from build123d import *

# Parameters (mm, degrees)
SKETCH_1_R          = 37.15
SKETCH_1_R_2        = 28
SKETCH_1_R_3        = 1.5
EXTRUDE_1_DEPTH     = 3
SKETCH_3_R          = 3
CUT_EXTRUDE_1_DEPTH = 2
CUT_EXTRUDE_START   = -0.5
SKETCH_4_R          = 37.15
CUT_EXTRUDE_2_DEPTH = 0.5


with BuildPart() as part:
    # 草图1 → 凸台-拉伸1 (new body)
    with BuildSketch(Plane(origin=(0, 0, 0), x_dir=(1, 0, 0), z_dir=(0, 1, 0))):
        with Locations(Location((0, 0, 0), (0, 0, 270))):
            Circle(SKETCH_1_R)
        with Locations(Location((0, 0, 0), (0, 0, 270))):
            Circle(SKETCH_1_R_2, mode=Mode.SUBTRACT)
        with Locations(Location((0, 34.825, 0), (0, 0, 270))):
            Circle(SKETCH_1_R_3, mode=Mode.SUBTRACT)
        with Locations(Location((-34.825, 0, 0), (0, 0, 270))):
            Circle(SKETCH_1_R_3, mode=Mode.SUBTRACT)
        with Locations(Location((0, -34.825, 0), (0, 0, 270))):
            Circle(SKETCH_1_R_3, mode=Mode.SUBTRACT)
        with Locations(Location((34.825, 0, 0), (0, 0, 270))):
            Circle(SKETCH_1_R_3, mode=Mode.SUBTRACT)
    extrude(amount=EXTRUDE_1_DEPTH)

    # 草图3 → 切除-拉伸1 (cut)
    with BuildSketch(Plane(origin=(0, 3, 0), x_dir=(1, 0, 0), z_dir=(0, 1, 0))):
        with Locations((0, 34.825)):
            Circle(SKETCH_3_R)
        with Locations((-34.825, 0)):
            Circle(SKETCH_3_R)
        with Locations((0, -34.825)):
            Circle(SKETCH_3_R)
        with Locations((34.825, 0)):
            Circle(SKETCH_3_R)
    extrude(amount=-CUT_EXTRUDE_1_DEPTH, mode=Mode.SUBTRACT)

    # 草图4 → 切除-拉伸2 (cut)
    with BuildSketch(Plane(origin=(0, 3, 0), x_dir=(1, 0, 0), z_dir=(0, 1, 0)).offset(CUT_EXTRUDE_START)):
        with Locations(Location((0, 0, 0), (0, 0, 93.02036647))):
            Circle(SKETCH_4_R)
    extrude(amount=CUT_EXTRUDE_2_DEPTH, mode=Mode.SUBTRACT)


solid = part.part
CAD build for the part. Positions are in the model's coordinates, mm. A direction names the side the tool comes from. Round coordinates to 2 decimals unless told otherwise and drop trailing zeros. Write each loop counter-clockwise with the first axis right and the second up, starting at its lowest first coordinate (ties: lowest second). Pieces come first, ordered by that corner, then holes.
(1) 3-axis set-ups, long thin cutter, end or side, ignore diameter. For faces 4 (the face through (0, 1, 33)), 5 (the face through (24, 2.5, -15)): which of +Z, -Z, +X, -X, +Y, -Y reach the whole face in a straight line?
(2) Drop flat-ended pins along their axis: P1, Ø4, axis at x = 0, z = -34.825, coming from the +Y side; P2, Ø1, axis at x = 7.5, y = 1.5, coming from the +Z side. Give the stop position or say it passes through.
(3) Slice it at C-C, the plane x = -11.5. Write the cut outline in (y, z).
(4) Probe line 1 along X through (y, z) = (0.35, 0) (3 decimals); line 2 along Z through (x, y) = (0, 2) (3 decimals); line 3 along X through (y, z) = (0.4, -0.5). List the from-to ranges inside material, lowest first.
(5) Mould opens along X. For faces 1 (the face through (11.159, 1.232, 35.434)), 2 (the face through (-25, 0, -14)), 3 (the face through (-0.913, 0.493, 33.635)) say: pulls with the +X half, pulls with the -X half, needs draft (parallel to the pull), parting line crosses it, or undercut.
(6) Slice it at A-A, the plane z = 0. Write the cut outline in (x, y) (3 decimals).
(7) Slice it at D-D, the plane z = -11. Write the cut outline in (x, y), and give its area (3 significant figures).
(8) Slice it at B-B, the plane x = 0. Write the cut outline in (y, z) (3 decimals).
From the geometry:
1. face 4: +Y
1. face 5: +Z, -Z, +X, -X, +Y
2. P1: stops at y = 1
2. P2: stops at z = 36.48
3. outline: (0, -35.33) - (2.5, -35.33) - (2.5, -25.53) - (0, -25.53) - close; (0, 25.53) - (2.5, 25.53) - (2.5, 35.33) - (0, 35.33) - close
4. line 1: x = -37.15 to -36.325, -33.325 to -28, 28 to 33.325, 36.325 to 37.15
4. line 2: z = -31.825 to -28, 28 to 31.825
4. line 3: x = -37.15 to -36.24, -33.41 to -28, 28 to 33.41, 36.24 to 37.15
5. face 1: parting line crosses it
5. face 2: needs draft
5. face 3: undercut
6. outline: (-37.15, 0) - (-36.325, 0) - (-36.325, 1) - (-37.15, 1) - close; (-33.325, 0) - (-28, 0) - (-28, 2.5) - (-31.825, 2.5) - (-31.825, 1) - (-33.325, 1) - close; (28, 0) - (33.325, 0) - (33.325, 1) - (31.825, 1) - (31.825, 2.5) - (28, 2.5) - close; (36.325, 0) - (37.15, 0) - (37.15, 1) - (36.325, 1) - close
7. outline: (-35.48, 0) - (-25.75, 0) - (-25.75, 2.5) - (-35.48, 2.5) - close; (25.75, 0) - (35.48, 0) - (35.48, 2.5) - (25.75, 2.5) - close
7. area: 48.7 mm2
8. outline: (0, -37.15) - (1, -37.15) - (1, -36.325) - (0, -36.325) - close; (0, -33.325) - (1, -33.325) - (1, -31.825) - (2.5, -31.825) - (2.5, -28) - (0, -28) - close; (0, 28) - (2.5, 28) - (2.5, 31.825) - (1, 31.825) - (1, 33.325) - (0, 33.325) - close; (0, 36.325) - (1, 36.325) - (1, 37.15) - (0, 37.15) - close
